Geometry: final body of the model. Coordinates: model frame, mm. Face numbers are marked on the shaded views. A direction names the side the tool comes from. Round coordinates to 2 decimals unless told otherwise and drop trailing zeros. Loops run counter-clockwise (first coordinate to the right, second up) from the corner with the lowest first, then second, coordinate; pieces in that order, holes last. Notation, with made-up numbers: M 57,54.5 L 95,54.5 A17 ccw 95,80.5 Z; hole C 80,-17.75 d7. An arc over 180 degrees is marked long. Answer as a JSON object with one key per item and string values.
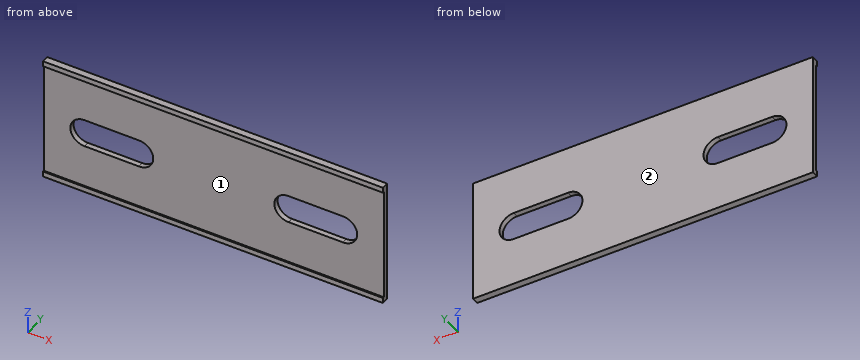
from build123d import *

# Parameters (mm, degrees)
BOSS_EXTRUDE1_DEPTH = 63.5
CUT_EXTRUDE1_DEPTH  = 68.763277548


with BuildPart() as part:
    # Sketch3 → Boss-Extrude1 (new body)
    with BuildSketch(Plane(origin=(0, 0, 0), x_dir=(0, 0, -1), z_dir=(1, 0, 0))):
        Polygon((0, 0), (23.622, 0), (23.622, -1.27), (22.606, -1.27), (22.606, -1.016), (1.016, -1.016), (1.016, -1.27), (0, -1.27), align=None)
    extrude(amount=BOSS_EXTRUDE1_DEPTH)

    # Sketch4 → Cut-Extrude1 (cut, through all)
    with BuildSketch(Plane(origin=(0, 0, 0), x_dir=(1, 0, 0), z_dir=(0, 1, 0))):
        with BuildLine():
            Line((7.62, 14.478), (17.78, 14.478))
            ThreePointArc((17.78, 14.478), (20.447, 11.811), (17.78, 9.144))
            Line((17.78, 9.144), (7.62, 9.144))
            ThreePointArc((7.62, 9.144), (4.953, 11.811), (7.62, 14.478))
        make_face()
        with BuildLine():
            Line((45.72, 9.144), (55.88, 9.144))
            ThreePointArc((55.88, 9.144), (58.547, 11.811), (55.88, 14.478))
            Line((55.88, 14.478), (45.72, 14.478))
            ThreePointArc((45.72, 14.478), (43.053, 11.811), (45.72, 9.144))
        make_face()
    extrude(amount=-CUT_EXTRUDE1_DEPTH, mode=Mode.SUBTRACT)


solid = part.part
1) Section query A-A (x = 9). Return the cut outline in (y, z).
Results:
{"outline": "M -1.27,-23.62 L 0,-23.62 L 0,-14.48 L -1.02,-14.48 L -1.02,-22.61 L -1.27,-22.61 Z; M -1.27,-1.02 L -1.02,-1.02 L -1.02,-9.14 L 0,-9.14 L 0,0 L -1.27,0 Z"}
2) Section query C-C (z = -11.75). Return the cut outline in (x, y).
Results:
{"outline": "M 0,-1.02 L 4.95,-1.02 L 4.95,0 L 0,0 Z; M 20.45,-1.02 L 43.05,-1.02 L 43.05,0 L 20.45,0 Z; M 58.55,-1.02 L 63.5,-1.02 L 63.5,0 L 58.55,0 Z"}
3) Section query B-B (y = -0.8). Return the cut outline in (x, z), and give its area (3 significant figures).
Results:
{"outline": "M 0,-23.62 L 63.5,-23.62 L 63.5,0 L 0,0 Z; hole M 7.62,-14.48 L 17.78,-14.48 A2.67 ccw 17.78,-9.14 L 7.62,-9.14 A2.67 ccw Z; hole M 45.72,-14.48 L 55.88,-14.48 A2.67 ccw 55.88,-9.14 L 45.72,-9.14 A2.67 ccw Z", "area": "1,350 mm2"}
4) Reachability of the marked faces 1 and 2 from +Z, -Z, +X, -X, +Y, -Y: full face, straight path, thin tool, end or side. Return the list, or none.
Results:
{"face 1": "+X, -X, -Y", "face 2": "+Z, -Z, +X, -X, +Y"}
5) Section query D-D (x = 38.5). Return the cut outline in (y, z).
Results:
{"outline": "M -1.27,-23.62 L 0,-23.62 L 0,0 L -1.27,0 L -1.27,-1.02 L -1.02,-1.02 L -1.02,-22.61 L -1.27,-22.61 Z"}
6) Ray query, line 1 (Z direction, x = 40, y = -1.2); line 2 (Z direction, x = 17.5, y = -0.85); line 3 (X direction, y = -0.9, z = -12.75). Return the intervals inside material, ascending.
Results:
{"line 1": "-23.62 to -22.61, -1.02 to 0", "line 2": "-23.62 to -14.48, -9.14 to 0", "line 3": "0 to 5.12, 20.28 to 43.22, 58.38 to 63.5"}
